Design review of the part built by this model. Coordinates are the model's own, in mm. Coordinates: 2 decimals unless noted, no trailing zeros. Loops run counter-clockwise (first coordinate to the right, second up) from the corner with the lowest first, then second, coordinate; pieces in that order, holes last.
Autodesk Inventor part; units mm, degrees
ref_plane "YZ Plane" through (0, 0, 0) normal (1, 0, 0) x (0, 1, 0)
ref_plane "XZ Plane" through (0, 0, 0) normal (0, 1, 0) x (-1, 0, 0)
ref_plane "XY Plane" through (0, 0, 0) normal (0, 0, 1) x (1, 0, 0)
sketch "Sketch1" plane through (0, 0, 0) normal (0, 0, 1) x (1, 0, 0)
  circle A0 centre (0, 0) radius 88.9
  circle A1 centre (0, 0) radius 117.475
  dimension "d0" = 177.8
  dimension "d2" = 28.575
extrude "Extrusion1" add sketch "Sketch1" along normal mid plane 12.7
sketch "Sketch2" plane through (0, 0, 6.35) normal (0, 0, 1) x (1, 0, 0)
  circle A0 centre (0, 0) radius 117.475
  line L0 (0, 0) -> (-47.625, 82.4889) construction
  line L1 (-164.465, 0) -> (164.465, 0)
  line L2 (0, -164.465) -> (0, 164.465)
  line L3 (-47.625, 82.4889) -> (-55.5625, 96.2371) construction
  dimension "d5" = 30
  dimension "d16" = 95.25
  dimension "d17" = 15.875
hole "Hole1" at (-47.625, 82.4889, 6.35) at (-55.5625, 96.2371, 6.35) direction (0, 0, -1) diameter 6.35 end through all
pattern_circular "Circular Pattern1" count 3 over 360 about axis through (0, 0, -10) along (0, 0, 1) of "Hole1"
properties part number "ring_top" material "Aluminum-6061"
Q1. The part is to be moulded in two halves that separate along Y. For faces 1 (the cylindrical face through (-93.224, 71.482, -0.089)), 2 (the flat face through (-27, -86, -6.35)), 3 (the cylindrical face through (114.225, 0.688, -0.089)), say which applies: pulls with the +Y half, pulls with the -Y half, needs draft (parallel to the pull), parting line crosses it, or undercut.
Q2. Take a section at A-A, the plane x = 0. Write out the cut boundary in (y, z) (3 decimals).
Q3. Take a section at C-C, the plane y = 25. Write out the cut boundary in (x, z).
Q4. For line 1 (Y direction, x = 0, z = -1.25) (3 decimals); line 2 (Y direction, x = -49.5, z = -4.5); line 3 (X direction, y = 1, z = 1.5), list the stretches that pass through material, from the lowest coordinate up.
Q5. Clearance check with a flat-ended pin moving along its axis: pin 1 Ø3 at (y, z) = (-15.5, 4.5) entering from -X. State where the tip first meets the part, or that it passes through.
Q6. Take a section at B-B, the plane z = -3.5. Give the number of separate pieces and of enclosed holes in the cut face, then the cut area to 3 significant figures.
Entries:
1. face 1: parting line crosses it
1. face 2: needs draft
1. face 3: undercut
2. outline: (-117.475, -6.35) - (-88.9, -6.35) - (-88.9, 6.35) - (-117.475, 6.35) - close; (88.9, -6.35) - (117.475, -6.35) - (117.475, 6.35) - (88.9, 6.35) - close
3. outline: (-114.78, -6.35) - (-85.31, -6.35) - (-85.31, 6.35) - (-114.78, 6.35) - close; (85.31, -6.35) - (114.78, -6.35) - (114.78, 6.35) - (85.31, 6.35) - close
4. line 1: y = -117.475 to -88.9, 88.9 to 117.475
4. line 2: y = -106.54 to -85.05, -79.93 to -73.84, 73.84 to 79.93, 85.05 to 106.54
4. line 3: x = -117.47 to -88.89, 88.89 to 92.24, 98.26 to 108.11, 114.14 to 117.47
5. pin 1: stops at x = -116.64
6. separate pieces: 1
6. enclosed holes: 7
6. area: 18,300 mm2
